from build123d import *

# Parameters (mm, degrees)
BOSS_EXTRUDE1_DEPTH = 5
SKETCH2_R           = 5
BOSS_EXTRUDE2_DEPTH = 3


with BuildPart() as part:
    # Sketch1 → Boss-Extrude1 (new body)
    with BuildSketch(Plane.XY):
        with BuildLine():
            Line((1, 0), (29, 0))
            ThreePointArc((29, 0), (29.707106781, 0.292893219), (30, 1))
            Line((30, 1), (30, 29))
            ThreePointArc((30, 29), (29.707106781, 29.707106781), (29, 30))
            Line((29, 30), (1, 30))
            ThreePointArc((1, 30), (0.292893219, 29.707106781), (0, 29))
            Line((0, 29), (0, 1))
            ThreePointArc((0, 1), (0.292893219, 0.292893219), (1, 0))
        make_face()
    extrude(amount=BOSS_EXTRUDE1_DEPTH)

    # Sketch2 → Boss-Extrude2 (add)
    with BuildSketch(Plane.XY.offset(5)):
        with Locations(Location((15, 15, 0), (0, 0, 180))):
            Circle(SKETCH2_R)
    extrude(amount=BOSS_EXTRUDE2_DEPTH)


solid = part.part
Design review of the part built by this model. Coordinates are the model's own, in mm. A direction names the side the tool comes from. Give positions to 0.01 mm unless a question says otherwise; leave off trailing zeros. Loops run counter-clockwise (first coordinate to the right, second up) from the corner with the lowest first, then second, coordinate; pieces in that order, holes last. Notation, with made-up numbers: (31.25, 27.5) - (82.25, 27.5) arc R22 cw to (82.25, 58.5) - close; hole circle Ø11 at (-16, 56.25). An arc over 180 degrees is marked (long way). Use CSV: the item, a comma, the result in double quotes. Start each with the question number.
1. Wall thickness on L1, parallel to Z at x = 20.25, y = 15; L2, parallel to X at y = 15.5, z = 6.75; L3, parallel to X at y = 12, z = 6.25: over which ranges is each line inside the solid? List them lowest first.
2. Insertion check: P1, Ø1.5, axis at x = 7, y = 7.5, coming from the +Z side. The pin has a flat end and moves straight along its axis. Give the tip position at first contact, or say it passes through.
3. Add section C-C (z = 6.25). State the section outline as (x, y) points, plus the area to 3 significant figures.
4. Add section A-A (y = 15). State the section outline as (x, z) points.
5. Add section D-D (x = 2.5). State the section outline as (y, z) points.
6. Machinability: for faces 1 (the flat face through (15, 30, 2)), 2 (the flat face through (11, 19, 5)), which of the approach directions +Z, -Z, +X, -X, +Y, -Y give a long, thin tool a straight path to every point of the face, cutting with its end or side? Answer none if there is none.
Results found:
1,L1,"z = 0 to 5"
1,L2,"x = 10.03 to 19.97"
1,L3,"x = 11 to 19"
2,P1,"stops at z = 5"
3,outline,"circle Ø10 at (15, 15)"
3,area,"78.5 mm²"
4,outline,"(0, 0) - (30, 0) - (30, 5) - (20, 5) - (20, 8) - (10, 8) - (10, 5) - (0, 5) - close"
5,outline,"(0, 0) - (30, 0) - (30, 5) - (0, 5) - close"
6,face 1,"+Z, -Z, +X, -X, +Y"
6,face 2,"+Z"
